The listing builds one solid part. Answer for the finished solid, in the listing's coordinates (mm). Face numbers are marked on the shaded views. A direction names the side the tool comes from. Coordinates: 2 decimals unless noted, no trailing zeros. Order: outer loops, then holes, each group sorted by start corner. A loop starts at its lowest first (then second) coordinate and runs counter-clockwise, first axis right, second up.
Autodesk Inventor part; units mm, degrees
ref_plane "YZ Plane" through (0, 0, 0) normal (1, 0, 0) x (0, 1, 0)
ref_plane "XZ Plane" through (0, 0, 0) normal (0, 1, 0) x (-1, 0, 0)
ref_plane "XY Plane" through (0, 0, 0) normal (0, 0, 1) x (1, 0, 0)
sketch "Sketch1" plane through (0, 0, 0) normal (0, 1, 0) x (-1, 0, 0)
  line L0 (0, 0) -> (1219.2, 0)
  line L1 (1219.2, 0) -> (1219.2, -1219.2)
  line L2 (1219.2, -1219.2) -> (0, -1219.2)
  line L3 (0, -1219.2) -> (0, 0)
  dimension "d0" = 1219.2
  dimension "d1" = 1219.2
extrude "Extrusion1" add sketch "Sketch1" along normal blind 25.4
sketch "Sketch2" plane through (0, 25.4, 0) normal (0, 1, 0) x (1, 0, 0)
  line L0 (-1107.5056, 119.0242) -> (-114.6697, 119.0242)
  line L1 (-114.6697, 119.0242) -> (-114.6697, 1047.9936)
  line L2 (-114.6697, 1047.9936) -> (-1107.5056, 1047.9936)
  line L3 (-1107.5056, 1047.9936) -> (-1107.5056, 119.0242)
  point P0 (0, 0)
extrude "Extrusion2" add sketch "Sketch2" along normal blind 1219.2
sketch "Sketch3" plane through (0, 1244.6, 0) normal (0, 1, 0) x (1, 0, 0)
  line L0 (-933.3238, 447.0665) -> (-759.1421, 447.0665)
  line L1 (-759.1421, 447.0665) -> (-759.1421, 688.0179)
  line L2 (-759.1421, 688.0179) -> (-933.3238, 688.0179)
  line L3 (-933.3238, 688.0179) -> (-933.3238, 447.0665)
  line L4 (-576.2513, 447.0665) -> (-480.4513, 447.0665)
  line L5 (-480.4513, 447.0665) -> (-480.4513, 545.7695)
  line L6 (-480.4513, 545.7695) -> (-576.2513, 545.7695)
  line L7 (-576.2513, 545.7695) -> (-576.2513, 447.0665)
  circle A0 centre (-528.3513, 705.4361) radius 55.5572
  circle A1 centre (-317.8817, 734.4664) radius 113.2181
  point P0 (0, 0)
extrude "Extrusion3" add sketch "Sketch3" along normal blind 76.2
sketch "Sketch4" plane through (-1107.5056, 25.4, -119.0242) normal (0, 0, 1) x (1, 0, 0)
  line L0 (30.4818, 1157.5843) -> (152.4572, 1157.5843)
  line L1 (152.4572, 1157.5843) -> (152.4572, 989.2087)
  line L2 (152.4572, 989.2087) -> (30.4818, 989.2087)
  line L3 (30.4818, 989.2087) -> (30.4818, 1157.5843)
  line L4 (0, 1219.2) -> (992.8359, 1219.2)
  line L5 (0, 0) -> (0, 1219.2)
  line L6 (233.6818, 1157.5843) -> (355.6572, 1157.5843)
  line L7 (355.6572, 1157.5843) -> (355.6572, 989.2087)
  line L8 (355.6572, 989.2087) -> (233.6818, 989.2087)
  line L9 (233.6818, 989.2087) -> (233.6818, 1157.5843)
  line L10 (436.8818, 1157.5843) -> (558.8572, 1157.5843)
  line L11 (558.8572, 1157.5843) -> (558.8572, 989.2087)
  line L12 (558.8572, 989.2087) -> (436.8818, 989.2087)
  line L13 (436.8818, 989.2087) -> (436.8818, 1157.5843)
  line L14 (640.0818, 1157.5843) -> (762.0572, 1157.5843)
  line L15 (762.0572, 1157.5843) -> (762.0572, 989.2087)
  line L16 (762.0572, 989.2087) -> (640.0818, 989.2087)
  line L17 (640.0818, 989.2087) -> (640.0818, 1157.5843)
  line L18 (843.2818, 1157.5843) -> (965.2572, 1157.5843)
  line L19 (965.2572, 1157.5843) -> (965.2572, 989.2087)
  line L20 (965.2572, 989.2087) -> (843.2818, 989.2087)
  line L21 (843.2818, 989.2087) -> (843.2818, 1157.5843)
  line L22 (30.4818, 852.7843) -> (152.4572, 852.7843)
  line L23 (152.4572, 852.7843) -> (152.4572, 684.4087)
  line L24 (152.4572, 684.4087) -> (30.4818, 684.4087)
  line L25 (30.4818, 684.4087) -> (30.4818, 852.7843)
  line L26 (233.6818, 852.7843) -> (355.6572, 852.7843)
  line L27 (355.6572, 852.7843) -> (355.6572, 684.4087)
  line L28 (355.6572, 684.4087) -> (233.6818, 684.4087)
  line L29 (233.6818, 684.4087) -> (233.6818, 852.7843)
  line L30 (436.8818, 852.7843) -> (558.8572, 852.7843)
  line L31 (558.8572, 852.7843) -> (558.8572, 684.4087)
  line L32 (558.8572, 684.4087) -> (436.8818, 684.4087)
  line L33 (436.8818, 684.4087) -> (436.8818, 852.7843)
  line L34 (640.0818, 852.7843) -> (762.0572, 852.7843)
  line L35 (762.0572, 852.7843) -> (762.0572, 684.4087)
  line L36 (762.0572, 684.4087) -> (640.0818, 684.4087)
  line L37 (640.0818, 684.4087) -> (640.0818, 852.7843)
  line L38 (843.2818, 852.7843) -> (965.2572, 852.7843)
  line L39 (965.2572, 852.7843) -> (965.2572, 684.4087)
  line L40 (965.2572, 684.4087) -> (843.2818, 684.4087)
  line L41 (843.2818, 684.4087) -> (843.2818, 852.7843)
  line L42 (30.4818, 547.9843) -> (152.4572, 547.9843)
  line L43 (152.4572, 547.9843) -> (152.4572, 379.6087)
  line L44 (152.4572, 379.6087) -> (30.4818, 379.6087)
  line L45 (30.4818, 379.6087) -> (30.4818, 547.9843)
  line L46 (233.6818, 547.9843) -> (355.6572, 547.9843)
  line L47 (355.6572, 547.9843) -> (355.6572, 379.6087)
  line L48 (355.6572, 379.6087) -> (233.6818, 379.6087)
  line L49 (233.6818, 379.6087) -> (233.6818, 547.9843)
  line L50 (436.8818, 547.9843) -> (558.8572, 547.9843)
  line L51 (558.8572, 547.9843) -> (558.8572, 379.6087)
  line L52 (558.8572, 379.6087) -> (436.8818, 379.6087)
  line L53 (436.8818, 379.6087) -> (436.8818, 547.9843)
  line L54 (640.0818, 547.9843) -> (762.0572, 547.9843)
  line L55 (762.0572, 547.9843) -> (762.0572, 379.6087)
  line L56 (762.0572, 379.6087) -> (640.0818, 379.6087)
  line L57 (640.0818, 379.6087) -> (640.0818, 547.9843)
  line L58 (843.2818, 547.9843) -> (965.2572, 547.9843)
  line L59 (965.2572, 547.9843) -> (965.2572, 379.6087)
  line L60 (965.2572, 379.6087) -> (843.2818, 379.6087)
  line L61 (843.2818, 379.6087) -> (843.2818, 547.9843)
  point P0 (1107.5056, -25.4)
  dimension "d10" = 203.2
  dimension "d13" = 304.8
extrude "Extrusion4" cut sketch "Sketch4" against normal blind 25.4
sketch "Sketch5" plane through (-1107.5056, 25.4, -1047.9936) normal (-1, 0, 0) x (0, 0, 1)
  line L0 (81.2848, 304.8) -> (865.1027, 304.8)
  line L1 (865.1027, 304.8) -> (865.1027, 0)
  line L2 (865.1027, 0) -> (81.2848, 0)
  line L3 (81.2848, 0) -> (81.2848, 304.8)
  line L4 (-171.2064, 0) -> (1047.9936, 0)
  point P0 (1047.9936, -25.4)
  dimension "d18" = 0
  dimension "d19" = 304.8
extrude "Extrusion5" cut sketch "Sketch5" against normal blind 609.6
equation "\"d1\" = d0"
properties part number "apartment_1" material "Wood (Oak)"
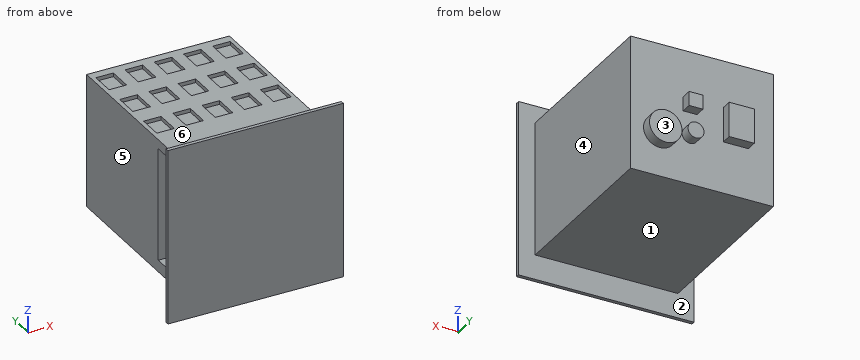
(1) The mould has two halves that part along Y. Classify the marked faces 1, 2 and 3: released by +Y, released by -Y, zero draft, split by the parting line, or undercut.
(2) Each of these flat-tipped pins is pushed along its axis until it touches: pin 1 Ø10 at (x, y) = (-1026.5, 554) entering from -Z; pin 2 Ø1.5 at (x, y) = (-497.5, 154) entering from +Z; pin 3 Ø3 at (y, z) = (291, -235.5) entering from -X; pin 4 Ø5 at (x, z) = (-956, -701) entering from -Y. Where does it stop, or does it pass through?
(3) Find section B-B (z = -414). Write down the section's boundary in (x, y).
(4) Consider line 1 (Y direction, x = -729, z = -711); line 2 (Z direction, x = -801, y = 583.5); line 3 (Z direction, x = -186, y = 1105.5). Determine where each line is inside the solid, lowest interval first.
(5) Find section C-C (y = 135). Write down the section's boundary in (x, z), and give its area (4 significant figures).
(6) Find section A-A (x = -705.5). Write down the section's boundary in (y, z).
(7) Find section D-D (y = 498.5). Write down the section's boundary in (x, z), and give its area (3 significant figures).
(8) For the marked faces 4, 5 and 6, determine the directions among +Z, -Z, +X, -X, +Y, -Y from which every point of the face is accessible in a straight line to the end or side of a thin tool.
Findings below:
1. face 1: zero draft
1. face 2: undercut
1. face 3: released by +Y
2. pin 1: stops at z = -1047.99
2. pin 2: stops at z = -119.02
2. pin 3: stops at x = -497.91
2. pin 4: stops at y = 0
3. outline: (-1219.2, 0) - (0, 0) - (0, 25.4) - (-114.67, 25.4) - (-114.67, 1244.6) - (-1107.51, 1244.6) - (-1107.51, 330.2) - (-497.91, 330.2) - (-497.91, 25.4) - (-1219.2, 25.4) - close
4. line 1: y = 0 to 25.4, 330.2 to 1244.6
4. line 2: z = -1047.99 to -119.02
4. line 3: z = -1047.99 to -144.42
5. outline: (-1107.51, -1047.99) - (-114.67, -1047.99) - (-114.67, -119.02) - (-1107.51, -119.02) - (-1107.51, -182.89) - (-497.91, -182.89) - (-497.91, -966.71) - (-1107.51, -966.71) - close
5. area: 444,500 mm2
6. outline: (0, -1219.2) - (25.4, -1219.2) - (25.4, -1047.99) - (1244.6, -1047.99) - (1244.6, -119.02) - (25.4, -119.02) - (25.4, 0) - (0, 0) - close; hole (25.4, -966.71) - (330.2, -966.71) - (330.2, -182.89) - (25.4, -182.89) - close
7. outline: (-1107.51, -1047.99) - (-114.67, -1047.99) - (-114.67, -119.02) - (-142.25, -119.02) - (-142.25, -144.42) - (-264.22, -144.42) - (-264.22, -119.02) - (-345.45, -119.02) - (-345.45, -144.42) - (-467.42, -144.42) - (-467.42, -119.02) - (-548.65, -119.02) - (-548.65, -144.42) - (-670.62, -144.42) - (-670.62, -119.02) - (-751.85, -119.02) - (-751.85, -144.42) - (-873.82, -144.42) - (-873.82, -119.02) - (-955.05, -119.02) - (-955.05, -144.42) - (-1077.02, -144.42) - (-1077.02, -119.02) - (-1107.51, -119.02) - close
7. area: 907,000 mm2
8. face 4: +Z, -Z, +X, +Y
8. face 5: +Z, -Z, -X, +Y
8. face 6: +Z, +X, -X, +Y
